```python
from build123d import *

# Parameters (mm, degrees)
SKETCH1_R               = 20
SKETCH1_R_2             = 5
BOSS_EXTRUDE1_DEPTH     = 20
SKETCH3_W               = 20
SKETCH3_H               = 30
SKETCH3_W_2             = 15
SKETCH3_H_2             = 20
SKETCH4_R               = 5
CUT_EXTRUDE1_DEPTH      = 1
CUT_EXTRUDE1_DEPTH_BACK = 21
SKETCH5_R               = 10
CUT_EXTRUDE2_DEPTH      = 1
CUT_EXTRUDE2_DEPTH_BACK = 17.5
SKETCH6_W               = 70
SKETCH6_H               = 30.026464272
SKETCH6_R               = 1.868076344
SKETCH6_W_2             = 20
SKETCH6_H_2             = 15
BOSS_EXTRUDE2_DEPTH     = 4


with BuildPart() as part:
    # Sketch1 → Boss-Extrude1 (new body)
    with BuildSketch(Plane.XY):
        Circle(SKETCH1_R)
        Circle(SKETCH1_R_2, mode=Mode.SUBTRACT)
    extrude(amount=BOSS_EXTRUDE1_DEPTH)

    # Sweep1: sweep along a path in Sketch2
    with BuildLine(Plane.XY) as sweep1_path:
        Line((0, 0), (-20, 0))
        ThreePointArc((-20, 0), (-27.90569415, 1.282917549), (-35, 5))
        ThreePointArc((-35, 5), (-84.088137289, 9.426274578), (-110, -32.5))
    # Sketch3 → Sweep1 (sweep)
    with BuildSketch(Plane(origin=(0, 0, 0), x_dir=(0, 0, -1), z_dir=(1, 0, 0))):
        with Locations((-10, 0)):
            Rectangle(SKETCH3_W, SKETCH3_H)
        with Locations((-10, 0)):
            Rectangle(SKETCH3_W_2, SKETCH3_H_2, mode=Mode.SUBTRACT)
    sweep(path=sweep1_path.line)

    # Mirror1: part across plane


with BuildPart() as part_1:
    add(part.part)
    add(part.part.mirror(Plane(origin=(0, 0, 0), x_dir=(0, 0, 1), z_dir=(1, 0, 0))))

    # Sketch4 → Cut-Extrude1 (cut, two sides)
    with BuildSketch(Plane.XY.offset(20)) as cut_extrude1_sk:
        Circle(SKETCH4_R)
    extrude(amount=CUT_EXTRUDE1_DEPTH, mode=Mode.SUBTRACT)
    extrude(cut_extrude1_sk.sketch, amount=-CUT_EXTRUDE1_DEPTH_BACK, mode=Mode.SUBTRACT)

    # Sketch5 → Cut-Extrude2 (cut, two sides)
    with BuildSketch(Plane(origin=(0, 0, 0), x_dir=(-1, 0, 0), z_dir=(0, 0, -1))) as cut_extrude2_sk:
        with Locations((-25, 0)):
            Circle(SKETCH5_R)
        with Locations((25, 0)):
            Circle(SKETCH5_R)
    extrude(amount=CUT_EXTRUDE2_DEPTH, mode=Mode.SUBTRACT)
    extrude(cut_extrude2_sk.sketch, amount=-CUT_EXTRUDE2_DEPTH_BACK, mode=Mode.SUBTRACT)

    # Sketch6 → Boss-Extrude2 (add)
    with BuildSketch(Plane.XZ.offset(32.5)):
        with Locations((110, 10)):
            Rectangle(SKETCH6_W, SKETCH6_H)
        with Locations((80, 22.5)):
            Circle(SKETCH6_R, mode=Mode.SUBTRACT)
        with Locations((140, 22.5)):
            Circle(SKETCH6_R, mode=Mode.SUBTRACT)
        with Locations((140, -2.5)):
            Circle(SKETCH6_R, mode=Mode.SUBTRACT)
        with Locations((80, -2.5)):
            Circle(SKETCH6_R, mode=Mode.SUBTRACT)
        with Locations((110, 10)):
            Rectangle(SKETCH6_W_2, SKETCH6_H_2, mode=Mode.SUBTRACT)
    extrude(amount=BOSS_EXTRUDE2_DEPTH)

    # Mirror2: part across plane


with BuildPart() as part_2:
    add(part_1.part)
    add(part_1.part.mirror(Plane(origin=(0, 0, 0), x_dir=(0, 0, 1), z_dir=(1, 0, 0))))


solid = part_2.part
```
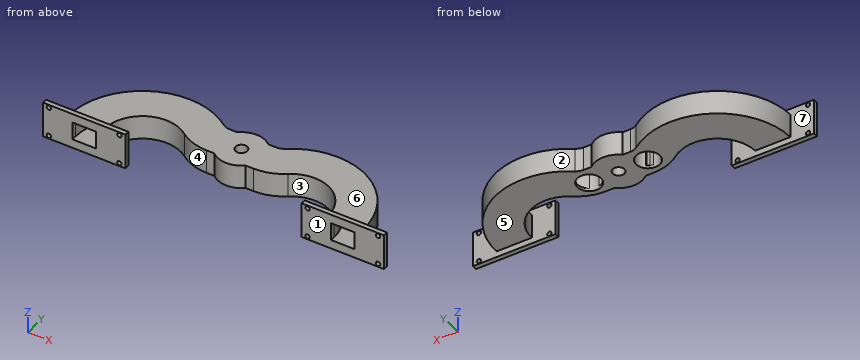
Verification items for the finished model (mm, model axes). Face numbers are marked on the shaded views. A direction names the side the tool comes from. Coordinates: 2 decimals unless noted, no trailing zeros. Loops run counter-clockwise (first coordinate to the right, second up) from the corner with the lowest first, then second, coordinate; pieces in that order, holes last. Notation, with made-up numbers: (-5, -25) - (24, -25) arc R9 cw to (24, -16) - close; hole circle Ø2 at (70, 83.5). An arc over 180 degrees is marked (long way). Answer as a JSON object with one key per item and string values.
(1) Mould release check, pull along X, two halves, no side actions. Record for the marked faces 6 and 7: pulls with the +X half, pulls with the -X half, needs draft (parallel to the pull), parting line crosses it, or undercut.
Response:
{"face 6": "needs draft", "face 7": "undercut"}
(2) Cross-section at B-B, the plane x = -114. Record the boundary of the cut face in (y, z).
Response:
{"outline": "(-36.5, -5.01) - (-32.5, -5.01) - (-32.5, 0) - (2.72, 0) - (2.72, 20) - (-32.5, 20) - (-32.5, 25.01) - (-36.5, 25.01) - (-36.5, 17.5) - (-7.07, 17.5) - (-7.07, 2.5) - (-36.5, 2.5) - close"}
(3) Scan lines: line 1 along Z through (x, y) = (-80, -35); line 2 along Y through (x, z) = (-81, 14.5); line 3 along X through (y, z) = (0, 10). Record each from-to range of solid material in increasing order.
Response:
{"line 1": "z = -5.01 to -4.37, -0.63 to 20.63, 24.37 to 25.01", "line 2": "y = -36.5 to -32.5, -6.11 to -0.25, 21.49 to 26.74", "line 3": "x = -115.78 to -109.8, -80.55 to -45.7, -15 to -5, 5 to 15, 45.7 to 80.55, 109.8 to 115.78"}
(4) Cross-section at A-A, the plane x = 0. Record the boundary of the cut face in (y, z), then the cut area to 3 significant figures.
Response:
{"outline": "(-20, 0) - (-5, 0) - (-5, 20) - (-20, 20) - close; (5, 0) - (20, 0) - (20, 20) - (5, 20) - close", "area": "600 mm²"}
(5) Access from +Z, -Z, +X, -X, +Y, -Y to the whole of each face (thin tool, end or side, straight path). Record for the marked faces 1, 2, 3, 4 and 5.
Response:
{"face 1": "+Z, -Z, +X, -X, -Y", "face 2": "+Z, -Z, +Y", "face 3": "+Z, -Z", "face 4": "+Z, -Z, -Y", "face 5": "-Z, +X, -X, +Y"}
(6) Go/stop test with flat-tipped pins: pin 1 Ø1.2 at (x, y) = (20.5, -9) entering from +Z; pin 2 Ø7.5 at (x, z) = (15, 8) entering from +Y; pin 3 Ø2 at (y, z) = (21, -0.5) entering from +X; pin 4 Ø2 at (x, z) = (-80, 22.5) entering from -Y. Record where each tip stops, or that it passes through.
Response:
{"pin 1": "stops at z = 20", "pin 2": "stops at y = 16.54", "pin 3": "stops at x = 95.65", "pin 4": "passes through"}
